```python
from build123d import *

# Parameters (mm, degrees)
F1_DEPTH = 428.625
F2_W     = 1.778
F2_H     = 214.3125
F3_DEPTH = 1.651
F4_R     = 3.175
F5_R     = 0.762
F6_DEPTH = 25.4


with BuildPart() as f1:
    # F0 (on Front) → F1 (new body)
    with BuildSketch(Plane.XZ):
        Polygon((0, 95.1738), (0, 96.8248), (-48.4124, 96.8248), (-48.4124, 0), (143.5862, 0), (143.5862, -95.1738), (96.8248, -95.1738), (96.8248, -96.8248), (145.2372, -96.8248), (145.2372, 1.651), (-46.7614, 1.651), (-46.7614, 95.1738), align=None)
    extrude(amount=F1_DEPTH)

    # F2 (on face) → F3 (cut)
    with BuildSketch(Plane(origin=(0, 0, 0), x_dir=(1, 0, 0), z_dir=(0, 0, -1))):
        with Locations((47.5869, 107.15625)):
            Rectangle(F2_W, F2_H)
        with BuildLine():
            Line((101.5619, 384.175), (101.5619, 406.4))
            ThreePointArc((101.5619, 406.4), (99.7020280605, 410.8901280605), (95.2119, 412.75))
            Line((95.2119, 412.75), (-0.0381, 412.75))
            ThreePointArc((-0.0381, 412.75), (-4.5282280605, 410.8901280605), (-6.3881, 406.4))
            Line((-6.3881, 406.4), (-6.3881, 384.175))
            ThreePointArc((-6.3881, 384.175), (-4.5282280605, 379.6848719395), (-0.0381, 377.825))
            Line((-0.0381, 377.825), (95.2119, 377.825))
            ThreePointArc((95.2119, 377.825), (99.7020280605, 379.6848719395), (101.5619, 384.175))
        make_face()
    extrude(amount=-F3_DEPTH, mode=Mode.SUBTRACT)

    # F4
    f4_edges = [f1.edges().sort_by_distance(p)[0] for p in [
        (48.4759, 0, 0.8255),
        (46.6979, 0, 0.8255),
    ]]
    fillet(f4_edges, radius=F4_R)

    # F5
    f5_edges = [f1.edges().sort_by_distance(p)[0] for p in [
        (46.6979, -214.3125, 0.8255),
        (48.4759, -214.3125, 0.8255),
    ]]
    fillet(f5_edges, radius=F5_R)

    # F2 (on face) → F6 (cut)
    with BuildSketch(Plane(origin=(0, 0, 0), x_dir=(1, 0, 0), z_dir=(0, 0, -1))):
        with Locations((47.5869, 107.15625)):
            Rectangle(F2_W, F2_H)
        with BuildLine():
            Line((101.5619, 384.175), (101.5619, 406.4))
            ThreePointArc((101.5619, 406.4), (99.7020280605, 410.8901280605), (95.2119, 412.75))
            Line((95.2119, 412.75), (-0.0381, 412.75))
            ThreePointArc((-0.0381, 412.75), (-4.5282280605, 410.8901280605), (-6.3881, 406.4))
            Line((-6.3881, 406.4), (-6.3881, 384.175))
            ThreePointArc((-6.3881, 384.175), (-4.5282280605, 379.6848719395), (-0.0381, 377.825))
            Line((-0.0381, 377.825), (95.2119, 377.825))
            ThreePointArc((95.2119, 377.825), (99.7020280605, 379.6848719395), (101.5619, 384.175))
        make_face()
    extrude(amount=-F6_DEPTH, mode=Mode.SUBTRACT)


solid = f1.part
```
CAD build for the part. Positions are in the model's coordinates, mm. A direction names the side the tool comes from. Round coordinates to 2 decimals unless told otherwise and drop trailing zeros. Write each loop counter-clockwise with the first axis right and the second up, starting at its lowest first coordinate (ties: lowest second). Pieces come first, ordered by that corner, then holes. Notation, with made-up numbers: (43.25, 60.25) - (67.25, 60.25) arc R19 cw to (67.25, 91.25) - close; hole circle Ø7 at (70, 4). An arc over 180 degrees is marked (long way). Return JSON: item names as keys, results as strings. Group by question number.
Item 1: Band-saw the part on C-C on y = -360.5. List the corners of the cut face in (x, z), plus the area to 3 significant figures.
Item 2: Band-saw the part on D-D on z = -13. List the corners of the cut face in (x, y) (3 decimals), plus the area to 3 significant figures.
Item 3: Band-saw the part on B-B on y = -187. List the corners of the cut face in (x, z).
Item 4: Probe probe 1 along Z at (x, y) = (129.5, -295); probe 2 along Z at (x, y) = (-38, -105); probe 3 along X at (y, z) = (-27, 1). List the from-to ranges inside material, lowest first.
Item 5: Flat gauge pins, fed straight in: pin 1 Ø0.5 at (y, z) = (-226.5, 96) entering from +X; pin 2 Ø14 at (x, y) = (-23, -114.5) entering from -Z; pin 3 Ø4 at (x, y) = (13, -135) entering from +Z. Where does each tip first touch, or does it go through?
Item 6: Band-saw the part on A-A on x = 57. List the corners of the cut face in (y, z) (3 decimals).
Item 7: 3-axis set-ups, long thin cutter, end or side, ignore diameter. For faces 1 (the face through (48, -428.625, 0.5)), 2 (the face through (-24, -211, 95.174)), 3 (the face through (143.586, -211, -47)): which of +Z, -Z, +X, -X, +Y, -Y reach the whole face in a straight line?
Item 8: Mould opens along Z. For faces 4 (the face through (121, -211, -96.825)), 5 (the face through (-46.761, -211, 48)), 6 (the face through (121, -211, -95.174)), 7 (the face through (-47, 0, 63)) say: +Z half, -Z half, draft (parallel to the pull), parting line (faces both ways), or undercut.
Resolved:
{
 "1": {"outline": "(-48.41, 0) - (143.59, 0) - (143.59, -95.17) - (96.82, -95.17) - (96.82, -96.82) - (145.24, -96.82) - (145.24, 1.65) - (-46.76, 1.65) - (-46.76, 95.17) - (0, 95.17) - (0, 96.82) - (-48.41, 96.82) - close", "area": "791 mm²"},
 "2": {"outline": "(143.586, -428.625) - (145.237, -428.625) - (145.237, 0) - (143.586, 0) - close", "area": "708 mm²"},
 "3": {"outline": "(-48.41, 0) - (46.7, 0) - (46.7, 1.65) - (-46.76, 1.65) - (-46.76, 95.17) - (0, 95.17) - (0, 96.82) - (-48.41, 96.82) - close; (48.48, 0) - (143.59, 0) - (143.59, -95.17) - (96.82, -95.17) - (96.82, -96.82) - (145.24, -96.82) - (145.24, 1.65) - (48.48, 1.65) - close"},
 "4": {"probe 1": "z = -96.82 to -95.17, 0 to 1.65", "probe 2": "z = 0 to 1.65, 95.17 to 96.82", "probe 3": "x = -48.41 to 46.7, 48.48 to 145.24"},
 "5": {"pin 1": "stops at x = 0", "pin 2": "stops at z = 0", "pin 3": "stops at z = 1.65"},
 "6": {"outline": "(-428.625, 0) - (-412.75, 0) - (-412.75, 1.651) - (-428.625, 1.651) - close; (-377.825, 0) - (0, 0) - (0, 1.651) - (-377.825, 1.651) - close"},
 "7": {"face 1": "+Z, -Z, +X, -X, -Y", "face 2": "+X, +Y, -Y", "face 3": "-X, +Y, -Y"},
 "8": {"face 4": "-Z half", "face 5": "undercut", "face 6": "undercut", "face 7": "draft"}
}
